Part model, mm, in its own coordinate system. A direction names the side the tool comes from. Round coordinates to 2 decimals unless told otherwise and drop trailing zeros. Order: outer loops, then holes, each group sorted by start corner. A loop starts at its lowest first (then second) coordinate and runs counter-clockwise, first axis right, second up. Notation, with made-up numbers: M 12,27.25 L 31,27.25 A6 cw 31,34.25 Z; hole C 86,45.5 d10. An arc over 180 degrees is marked long. One line per question, with ' | ' between items.
Autodesk Inventor part; units mm, degrees
ref_plane "YZ Plane" through (0, 0, 0) normal (1, 0, 0) x (0, 1, 0)
ref_plane "XZ Plane" through (0, 0, 0) normal (0, 1, 0) x (-1, 0, 0)
ref_plane "XY Plane" through (0, 0, 0) normal (0, 0, 1) x (1, 0, 0)
sketch "Sketch1" plane through (0, 0, 0) normal (0, 0, 1) x (1, 0, 0)
  circle A0 centre (0, 0) radius 2.2451
extrude "Extrusion1" add sketch "Sketch1" against normal blind 5.08
sketch "Sketch2" plane through (0, 0, 0) normal (0, 0, 1) x (1, 0, 0)
  circle A0 centre (0, 0) radius 2.2451
  line L0 (2.2451, 1.3979) -> (2.3331, -1.2453)
  line L1 (2.3331, -1.2453) -> (0.0881, -2.6432)
  line L2 (0.0881, -2.6432) -> (-2.2451, -1.3979)
  line L3 (-2.2451, -1.3979) -> (-2.3331, 1.2453)
  line L4 (-2.3331, 1.2453) -> (-0.0881, 2.6432)
  line L5 (-0.0881, 2.6432) -> (2.2451, 1.3979)
extrude "Extrusion2" add sketch "Sketch2" along normal blind 0.381 and the other way blind 2.54 contours A0 | L0 L1 L2 L3 L4 L5
sketch "Sketch3" plane through (0, 0, 0.381) normal (0, 0, 1) x (1, 0, 0)
  circle A0 centre (0, 0) radius 3.5571
extrude "Extrusion3" add sketch "Sketch3" along normal blind 3.81
sketch "Sketch4" plane through (0, 0, 4.191) normal (0, 0, 1) x (1, 0, 0)
  circle A0 centre (0, 0) radius 2.5038
extrude "Extrusion4" add sketch "Sketch4" along normal blind 2.54
properties part number "SC DC MOTOR"
1) Saw through at D-D (z = -3). List the corners of the cut face in (x, y).
The answers:
outline: C 0,0 d4.49
2) Saw through at C-C (z = 6). List the corners of the cut face in (x, y), plus the area to 3 significant figures.
The answers:
outline: C 0,0 d5.01 | area: 19.7 mm²
3) Saw through at A-A (x = -0.25). List the corners of the cut face in (y, z), plus the area to 3 significant figures.
The answers:
outline: M -3.55,0.38 L -2.46,0.38 L -2.46,-2.54 L -2.23,-2.54 L -2.23,-5.08 L 2.23,-5.08 L 2.23,-2.54 L 2.54,-2.54 L 2.54,0.38 L 3.55,0.38 L 3.55,4.19 L 2.49,4.19 L 2.49,6.73 L -2.49,6.73 L -2.49,4.19 L -3.55,4.19 Z | area: 65.6 mm²
4) Saw through at B-B (y = 1). List the corners of the cut face in (x, z), plus the area to 3 significant figures.
The answers:
outline: M -3.41,0.38 L -2.32,0.38 L -2.32,-2.54 L -2.01,-2.54 L -2.01,-5.08 L 2.01,-5.08 L 2.01,-2.54 L 2.26,-2.54 L 2.26,0.38 L 3.41,0.38 L 3.41,4.19 L 2.3,4.19 L 2.3,6.73 L -2.3,6.73 L -2.3,4.19 L -3.41,4.19 Z | area: 61.3 mm²
5) Drop flat-ended pins along their axis: pin 1 (3 mm diameter, centred on x = -0.5, z = 2, fed in from -Y); pin 2 (3 mm diameter, centred on x = 2.5, z = -2, fed in from +Y). Give the stop position or say it passes through.
The answers:
pin 1: stops at y = -3.56 | pin 2: stops at y = 2.06
6) Probe line 1 (Z direction, x = -2.75, y = 2); line 2 (Z direction, x = -2, y = 1.25); line 3 (Y direction, x = 0.25, z = -3). List the from-to ranges inside material, lowest first. Write a range as [from, to].
The answers:
line 1: z = [0.38, 4.19] | line 2: z = [-2.54, 6.73] | line 3: y = [-2.23, 2.23]
7) Which spindle directions (+Z, -Z, +X, -X, +Y, -Y) get a long thin tool onto all of the face, cutting with end or side? Do faces 1 (the face through (1.23, -1.93, -1.06)), 2 (the face through (2.141, 0.674, -3.792)), 3 (the face through (-1.23, 1.93, -1.06)), 4 (the face through (2, -2, 4.191)). Say none if no direction does.
The answers:
face 1: -Z, +X, -Y | face 2: -Z | face 3: -Z, -X, +Y | face 4: +Z
